Check sheet for the modelled part. Datum: model origin and axes. Units: mm. A direction names the side the tool comes from. Give positions to 0.01 mm unless a question says otherwise; leave off trailing zeros. Order: outer loops, then holes, each group sorted by start corner. A loop starts at its lowest first (then second) coordinate and runs counter-clockwise, first axis right, second up.
Item 1: Access from +Z, -Z, +X, -X, +Y, -Y to the whole of each face (thin tool, end or side, straight path). Record for faces 1 (the flat face through (0, 25.4, 0)), 2 (the cylindrical face through (24.04, 12.8, -23.75)).
Item 2: Release check for a two-part mould opening along Z. For faces 3 (the flat face through (17.78, 15, -27)), 4 (the flat face through (30.48, 13, -26)) record: released by +Z, released by -Z, zero draft, split by the parting line, or undercut.
Item 3: Sectioned sample at A-A on z = 0. Record the boundary of the cut face in (x, y).
Item 4: Sectioned sample at B-B on y = 12.7. Record the boundary of the cut face in (x, z).
Item 5: Sectioned sample at C-C on y = 2.5. Record the boundary of the cut face in (x, z), and give its area (3 significant figures).
Item 6: Material ranges on line 1 along Z through (x, y) = (25.5, 12.75); line 2 along Z through (x, y) = (-17, 16); line 3 along X through (y, z) = (2.5, -6), recorded low to high.
Item 7: Sectioned sample at D-D on y = 22. Record the boundary of the cut face in (x, z), and give its area (3 significant figures).
Item 8: Gauge pin test, flat ends, axial feed: P1, Ø3, axis at x = -10.5, y = 18.5, coming from the +Z side; P2, Ø4, axis at x = -5, y = 15.5, coming from the +Z side; P3, Ø12, axis at x = -22.5, z = 19.5, coming from the +Y side; P4, Ø1, axis at x = 10.5, z = -12, coming from the -Y side. Record the tip position at first contact, or that the pin passes through.
from build123d import *

# Parameters (mm, degrees)
SKETCH1_R           = 29.21
BOSS_EXTRUDE1_DEPTH = 25.4
FILLET1_R           = 11.43
SKETCH2_R           = 3.175
BOSS_EXTRUDE2_DEPTH = 17.78
SKETCH3_R           = 2.286
BOSS_EXTRUDE3_DEPTH = 12.7


with BuildPart() as part:
    # Sketch1 → Boss-Extrude1 (new body)
    with BuildSketch(Plane(origin=(0, 0, 0), x_dir=(1, 0, 0), z_dir=(0, 1, 0))):
        with Locations(Location((0, 0, 0), (0, 0, 270))):
            Circle(SKETCH1_R)
    extrude(amount=BOSS_EXTRUDE1_DEPTH)

    # Fillet1
    fillet1_edges = [part.edges().sort_by_distance(p)[0] for p in [
        (0, 0, -29.21),
        (0, 25.4, -29.21),
    ]]
    fillet(fillet1_edges, radius=FILLET1_R)

    # Sketch2 → Boss-Extrude2 (add)
    with BuildSketch(Plane(origin=(0, 0, 0), x_dir=(0, 0, -1), z_dir=(1, 0, 0))):
        with Locations((26.035, 12.7)):
            Circle(SKETCH2_R)
    extrude(amount=BOSS_EXTRUDE2_DEPTH)

    # Sketch3 → Boss-Extrude3 (add)
    with BuildSketch(Plane(origin=(17.78, 0, 0), x_dir=(0, 0, -1), z_dir=(1, 0, 0))):
        with Locations((26.035, 12.7)):
            Circle(SKETCH3_R)
    extrude(amount=BOSS_EXTRUDE3_DEPTH)


solid = part.part
Report:
1. face 1: +Z, -Z, +X, -X, +Y
1. face 2: +X
2. face 3: undercut
2. face 4: zero draft
3. outline: (-29.21, 11.43) arc R11.43 ccw to (-17.78, 0) - (17.78, 0) arc R11.43 ccw to (29.21, 11.43) - (29.21, 13.97) arc R11.43 ccw to (17.78, 25.4) - (-17.78, 25.4) arc R11.43 ccw to (-29.21, 13.97) - close
4. outline: (0, -29.21) - (17.78, -29.21) - (17.78, -28.32) - (30.48, -28.32) - (30.48, -23.75) - (17.78, -23.75) - (17.78, -23.18) arc R29.21 ccw (long way) to start
5. outline: circle Ø49.83 at (0, 0)
5. area: 1,950 mm2
6. line 1: z = -28.32 to -23.75, -14.25 to 14.25
6. line 2: z = -23.53 to 23.53
6. line 3: x = -24.18 to 24.18
7. outline: circle Ø51.83 at (0, 0)
7. area: 2,110 mm2
8. P1: stops at z = 27.07
8. P2: stops at z = 29.02
8. P3: stops at y = 23.7
8. P4: stops at y = 0
